Autodesk Inventor part; units mm, degrees
ref_plane "YZ Plane" through (0, 0, 0) normal (1, 0, 0) x (0, 1, 0)
ref_plane "XZ Plane" through (0, 0, 0) normal (0, 1, 0) x (-1, 0, 0)
ref_plane "XY Plane" through (0, 0, 0) normal (0, 0, 1) x (1, 0, 0)
sketch "スケッチ1" plane through (0, 0, 0) normal (0, 1, 0) x (-1, 0, 0)
  line L0 (0, 0) -> (-23, 0)
  line L1 (-23, 0) -> (-23, -12.5)
  line L2 (-23, -12.5) -> (0, -12.5)
  line L3 (0, -12.5) -> (0, 0)
  dimension "d0" = 23
  dimension "d1" = 12.5
extrude "押し出し1" add sketch "スケッチ1" along normal blind 15
sketch "スケッチ2" plane through (0, 15, 0) normal (0, 1, 0) x (1, 0, 0)
  line L0 (23, 0) -> (23, 12.5)
  line L1 (23, 12.5) -> (0, 12.5)
  line L2 (0, 12.5) -> (0, 0)
  line L3 (0, 0) -> (23, 0)
  line L4 (-4, 0) -> (27, 0)
  line L5 (27, 0) -> (27, 12.5)
  line L6 (27, 12.5) -> (-4, 12.5)
  line L7 (-4, 12.5) -> (-4, 0)
  dimension "d4" = 4
  dimension "d5" = 4
extrude "押し出し2" add sketch "スケッチ2" along normal blind 2.5
sketch "スケッチ3" plane through (0, 17.5, 0) normal (0, 1, 0) x (1, 0, 0)
  line L0 (-4, 0) -> (27, 0)
  line L1 (27, 12.5) -> (-4, 12.5)
  line L2 (0, 12.5) -> (0, 0)
  line L3 (23, 0) -> (23, 12.5)
extrude "押し出し3" add sketch "スケッチ3" along normal blind 4
sketch "スケッチ4" plane through (0, 21.5, 0) normal (0, 1, 0) x (1, 0, 0)
  line L0 (23, 12.5) -> (0, 12.5)
  line L1 (0, 12.5) -> (0, 0)
  line L2 (0, 0) -> (23, 0)
  circle A0 centre (6.25, 6.25) radius 6.25
extrude "押し出し4" add sketch "スケッチ4" along normal blind 4.3 contours A0
sketch "スケッチ5" plane through (6.25, 25.8, -6.25) normal (0, 1, 0) x (1, 0, 0)
  circle A0 centre (0, 0) radius 6.25
  point P0 (-6.25, -6.25)
hole "穴1" at (6.25, 25.8, -6.25) direction (0, -1, 0) diameter 3 end through all
equation "\"d5\" = d4"
properties part number "ServoMotor_10g"
Build history of the part. All positions in model axes, mm. A direction names the side the tool comes from. Round coordinates to 2 decimals unless told otherwise and drop trailing zeros. Write each loop counter-clockwise with the first axis right and the second up, starting at its lowest first coordinate (ties: lowest second). Pieces come first, ordered by that corner, then holes. Notation, with made-up numbers: M -8.5,-15 L 4.5,-15 A3 ccw 4.5,-11 Z; hole C 14,-0.75 d6. An arc over 180 degrees is marked long. Answer as a JSON object with one key per item and string values. Group by question number.
(1) Drill centre lines: L1, parallel to X at y = 10.25, z = -6.25; L2, parallel to Z at x = 6.25, y = 13; L3, parallel to Y at x = -1.5, z = -6. Where is each one in solid material? Low to high.
(2) Cut at B-B (y = 19). Give the cut face in (x, z), and give its area (3 significant figures).
(3) Cut at D-D (x = 19). Give the cut face in (y, z).
(4) Cut at C-C (z = -9). Give the cut face in (x, y), and give its area (3 significant figures).
(5) Cut at A-A (z = -5.5). Give the cut face in (x, y).
(6) Mould opens along Y. For faces 1 (the flat face through (0, 7, -6)), 2 (the flat face through (-2, 17.5, -6)), 3 (the flat face through (-2, 15, -6)) say: pulls with the +Y half, pulls with the -Y half, needs draft (parallel to the pull), parting line crosses it, or undercut.
(7) Which spindle directions (+Z, -Z, +X, -X, +Y, -Y) get a long thin tool onto all of the face, cutting with end or side? Do faces 4 (the cylindrical face through (0.006, 23.62, -5.975)), 5 (the flat face through (0, 19, -6)), 6 (the flat face through (23, 19, -6)). Say none if no direction does.
(8) Flat gauge pins, fed straight in: pin 1 (3 mm diameter, centred on x = -2.5, z = -4.5, fed in from +Y); pin 2 (3 mm diameter, centred on x = 25.5, z = -4, fed in from -Y); pin 3 (4 mm diameter, centred on y = 21.5, z = -4, fed in from -X). Where does each tip first touch, or does it go through?
Responses:
{
 "1": {"L1": "x = 0 to 4.75, 7.75 to 23", "L2": "z = -12.5 to -7.75, -4.75 to 0", "L3": "y = 15 to 17.5"},
 "2": {"outline": "M 0,-12.5 L 23,-12.5 L 23,0 L 0,0 Z; hole C 6.25,-6.25 d3", "area": "280 mm2"},
 "3": {"outline": "M 0,-12.5 L 21.5,-12.5 L 21.5,0 L 0,0 Z"},
 "4": {"outline": "M -4,15 L 0,15 L 0,0 L 23,0 L 23,15 L 27,15 L 27,17.5 L 23,17.5 L 23,21.5 L 11.86,21.5 L 11.86,25.8 L 0.64,25.8 L 0.64,21.5 L 0,21.5 L 0,17.5 L -4,17.5 Z", "area": "563 mm2"},
 "5": {"outline": "M -4,15 L 0,15 L 0,0 L 4.95,0 L 4.95,25.8 L 0.05,25.8 L 0.05,21.5 L 0,21.5 L 0,17.5 L -4,17.5 Z; M 7.55,0 L 23,0 L 23,15 L 27,15 L 27,17.5 L 23,17.5 L 23,21.5 L 12.45,21.5 L 12.45,25.8 L 7.55,25.8 Z"},
 "6": {"face 1": "needs draft", "face 2": "pulls with the +Y half", "face 3": "pulls with the -Y half"},
 "7": {"face 4": "+Y", "face 5": "+Z, -Z, -X, +Y", "face 6": "+Z, -Z, +X, +Y"},
 "8": {"pin 1": "stops at y = 17.5", "pin 2": "stops at y = 15", "pin 3": "stops at x = 0"}
}
